Autodesk Inventor part; units mm, degrees
ref_plane "YZ Plane" through (0, 0, 0) normal (1, 0, 0) x (0, 1, 0)
ref_plane "XZ Plane" through (0, 0, 0) normal (0, 1, 0) x (-1, 0, 0)
ref_plane "XY Plane" through (0, 0, 0) normal (0, 0, 1) x (1, 0, 0)
sketch "Sketch1" plane through (0, 0, 0) normal (0, 0, 1) x (1, 0, 0)
  arc A0 (6.3485, -145.912) -> (6.35, 145.9119) centre (0, 0) ccw
  line L0 (6.35, -150.9919) -> (6.35, -151.13)
  line L1 (6.35, 145.9119) -> (6.35, 168.7906)
  line L2 (0, 0) -> (0, 200.5264) construction
  line L3 (6.35, 145.9119) -> (6.35, 150.9919) construction
  line L4 (6.35, 150.9919) -> (-25.4, 150.9919)
  line L5 (-25.4, 150.9919) -> (-25.4, 161.1519)
  line L6 (-25.4, 161.1519) -> (6.35, 161.1519)
  line L7 (0, -146.05) -> (0, 0) construction
  line L8 (168.91, 0) -> (168.91, -76.2)
  line L9 (168.91, -76.2) -> (150.7453, -76.2)
  line L10 (0, 0) -> (0, -63.5) construction
  line L11 (0, -63.5) -> (158.75, -63.5) construction
  line L12 (158.75, -58.7375) -> (163.83, -58.7375)
  line L13 (163.83, -58.7375) -> (163.83, -68.2625)
  line L14 (163.83, -68.2625) -> (153.67, -68.2625)
  line L15 (153.67, -68.2625) -> (153.67, -58.7375)
  line L16 (153.67, -58.7375) -> (158.75, -58.7375)
  arc A1 (6.3485, -168.7907) -> (150.7453, -76.2) centre (0, 0) ccw
  line L17 (6.35, 161.1519) -> (-6.35, 161.1519) construction
  line L18 (-6.35, 161.1519) -> (-6.35, 168.7906) construction
  line L19 (0, -146.05) -> (0, -151.13) construction
  line L20 (6.3485, -151.13) -> (25.4, -151.13)
  line L21 (25.4, -151.13) -> (25.4, -161.29)
  line L22 (25.4, -161.29) -> (6.3485, -161.29)
  arc A2 (168.91, 0) -> (6.35, 168.7906) centre (0, 0) ccw
  line L23 (0, -146.05) -> (6.3485, -145.912) construction
  line L24 (6.3485, -145.912) -> (6.3485, -151.13)
  line L25 (6.3485, -161.29) -> (6.3485, -168.7907)
  line L26 (6.3485, -145.912) -> (6.3485, -151.13) construction
  line L27 (6.3485, -161.29) -> (6.3485, -184.4747) construction
  line L28 (0, 0) -> (762, -1319.8227) construction
  line L29 (0, 0) -> (1524, 0) construction
  line L30 (0, 0) -> (158.4844, 274.503) construction
  line L31 (0, 0) -> (316.9688, 0) construction
  line L32 (76.2, -131.9823) -> (78.9496, -130.3948)
  line L33 (78.9496, -130.3948) -> (82.1246, -135.894)
  line L34 (82.1246, -135.894) -> (76.6254, -139.069)
  line L35 (76.6254, -139.069) -> (73.4504, -133.5698)
  line L36 (73.4504, -133.5698) -> (76.2, -131.9823)
  line L37 (152.4, 0) -> (152.4, -3.175)
  line L38 (152.4, -3.175) -> (158.75, -3.175)
  line L39 (158.75, -3.175) -> (158.75, 3.175)
  line L40 (158.75, 3.175) -> (152.4, 3.175)
  line L41 (152.4, 3.175) -> (152.4, -3.175)
  line L42 (73.4504, 133.5698) -> (76.6254, 139.069)
  line L43 (76.6254, 139.069) -> (82.1246, 135.894)
  line L44 (82.1246, 135.894) -> (78.9496, 130.3948)
  line L45 (78.9496, 130.3948) -> (73.4504, 133.5698)
  line L46 (168.91, -76.2) -> (168.91, -50.8) construction
  line L47 (168.91, -50.8) -> (152.4, -50.8)
  line L48 (152.4, -50.8) -> (168.91, 0)
  line L49 (168.91, -50.8) -> (168.91, 0)
  point P0 (6.35, -145.9119)
  point P1 (0.0447, 168.91)
  point P2 (6.3947, 145.9099)
  dimension "d51" = 292.1
  dimension "d72" = 6.35
  dimension "d73" = 5.08
  dimension "d75" = 31.75
  dimension "d76" = 10.16
  dimension "d82" = 76.2
  dimension "d86" = 63.5
  dimension "d87" = 158.75
  dimension "d89" = 4.7625
  dimension "d90" = 5.08
  dimension "d91" = 9.525
  dimension "d92" = 10.16
  dimension "d93" = 4.7625
  dimension "d100" = 12.7
  dimension "d101" = 5.08
  dimension "d103" = 25.4
  dimension "d104" = 10.16
  dimension "d105" = 6.35
  dimension "d106" = 7.5007
  dimension "d107" = 25.4
  dimension "d113" = 1524
  dimension "d114" = 60
  dimension "d115" = 60
  dimension "d121" = 3.175
  dimension "d122" = 6.35
  dimension "d123" = 152.4
  dimension "d124" = 6.35
  dimension "d125" = 3.175
  dimension "d126" = 6.35
  dimension "d127" = 6.35
  dimension "d128" = 152.4
  dimension "d130" = 6.35
  dimension "d131" = 6.35
  dimension "d132" = 6.35
  dimension "d133" = 3.175
  dimension "d134" = 152.4
  dimension "d139" = 25.4
  dimension "d140" = 71.996
extrude "Extrusion21" add sketch "Sketch1" along normal blind 6.35 contours A0 L1 A2 L48 L47 L8 L9 A1 L25 L22 L21 L20 L0 L24 | L4 L5 L6 L1
properties part number "TopHoopSection_v4"
Source: CAD feature listing. Evaluate the final solid. Frame: model axes, mm. A direction names the side the tool comes from. Coordinates: 2 decimals unless noted, no trailing zeros. Write each loop counter-clockwise with the first axis right and the second up, starting at its lowest first coordinate (ties: lowest second). Pieces come first, ordered by that corner, then holes. Notation, with made-up numbers: M 80,57 L 111,57 A18 ccw 111,84 Z; hole C 16.5,72 d7. An arc over 180 degrees is marked long. Use a Markdown table: item, result.
1) Ray query, L1, parallel to Y at x = 12, z = 0.5; L2, parallel to Y at x = 90, z = 2.5; L3, parallel to Y at x = 100, z = 2.5. Return the intervals inside material, ascending.
Conclusion:
| item | result |
|---|---|
| L1 | y = -168.48 to -161.29, -151.13 to -145.56, 145.56 to 168.48 |
| L2 | y = -142.94 to -115.02, 115.02 to 142.94 |
| L3 | y = -136.13 to -106.45, 106.45 to 136.13 |
2) Mould query, pull axis X, two halves, no side actions, for faces 1 (the flat face through (-9, 150.992, 3)), 2 (the cylindrical face through (120.397, 118.47, 3.131)), 3 (the flat face through (152.4, 0, 3)). Classes: pulls with the +X half, pulls with the -X half, needs draft (parallel to the pull), parting line crosses it, or undercut.
Conclusion:
| item | result |
|---|---|
| face 1 | needs draft |
| face 2 | pulls with the +X half |
| face 3 | undercut |
3) First-contact query: pin 1 Ø3 at (x, z) = (72.5, 2.5) entering from -Y; pin 2 Ø3 at (x, z) = (-4, 3) entering from -Y; pin 3 Ø1.9 at (y, z) = (-64.5, 2) entering from -X. Flat tips, straight axial feed; report the tip coordinate or a pass-through.
Conclusion:
| item | result |
|---|---|
| pin 1 | stops at y = -153.26 |
| pin 2 | stops at y = 150.99 |
| pin 3 | stops at x = 130.56 |
4) Section A-A, the plane z = 3.25. Give the number of separate pieces and of enclosed holes in the cut face, then the cut area to 3 significant figures.
Conclusion:
| item | result |
|---|---|
| separate pieces | 1 |
| enclosed holes | 4 |
| area | 11,000 mm^2 |
5) Reachability of faces 4 (the flat face through (6.35, 165, 3)), 5 (the flat face through (25.4, -156, 3)), 6 (the flat face through (6.348, -165, 3)), 7 (the flat face through (160, -76.2, 3)), 8 (the flat face through (153.67, -64, 3)) from +Z, -Z, +X, -X, +Y, -Y: full face, straight path, thin tool, end or side. Return the list, or none.
Conclusion:
| item | result |
|---|---|
| face 4 | +Z, -Z, -X, +Y |
| face 5 | +Z, -Z, -X |
| face 6 | +Z, -Z, -X, -Y |
| face 7 | +Z, -Z, +X, -Y |
| face 8 | +Z, -Z |
6) Section D-D, the plane y = -34. Output: boundary loops of the cut face in (x, z), then the cut area to 3 significant figures.
Conclusion:
| item | result |
|---|---|
| outline | M 142.04,0 L 157.86,0 L 157.86,6.35 L 142.04,6.35 Z |
| area | 100 mm^2 |
7) Section B-B, the plane x = 17. Output: boundary loops of the cut face in (y, z), then the cut area to 3 significant figures.
Conclusion:
| item | result |
|---|---|
| outline | M -168.05,0 L -161.29,0 L -161.29,6.35 L -168.05,6.35 Z; M -151.13,0 L -145.06,0 L -145.06,6.35 L -151.13,6.35 Z; M 145.06,0 L 168.05,0 L 168.05,6.35 L 145.06,6.35 Z |
| area | 228 mm^2 |
8) Section C-C, the plane x = 37. Output: boundary loops of the cut face in (y, z).
Conclusion:
| item | result |
|---|---|
| outline | M -164.81,0 L -141.29,0 L -141.29,6.35 L -164.81,6.35 Z; M 141.29,0 L 164.81,0 L 164.81,6.35 L 141.29,6.35 Z |
